```python
from build123d import *

# Parameters (mm, degrees)
F1_DEPTH       = 180
F3_D           = 4.5
F3_CBORE_D     = 8.5
F3_CBORE_DEPTH = 5.5


with BuildPart() as f1:
    # F0 (on Right) → F1 (new body)
    with BuildSketch(Plane.YZ):
        with BuildLine():
            Line((-6.8, 0), (6.8, 0))
            Line((6.8, 0), (7.5, 0.7))
            Line((7.5, 0.7), (7.5, 3.699439))
            Line((7.5, 3.699439), (4.799805, 6.399634))
            Line((4.799805, 6.399634), (4.799805, 8.409149))
            Line((4.799805, 8.409149), (5.200758, 8.810103))
            ThreePointArc((5.200758, 8.810103), (5.668922, 9.789262), (6.648081, 10.257425))
            Line((6.648081, 10.257425), (7.5, 11.109345))
            Line((7.5, 11.109345), (7.5, 12.449454))
            Line((7.5, 12.449454), (6.634491, 13.314965))
            ThreePointArc((6.634491, 13.314965), (5.668922, 13.781617), (5.20227, 14.747186))
            Line((5.20227, 14.747186), (4.949456, 15))
            Line((4.949456, 15), (-4.949456, 15))
            Line((-4.949456, 15), (-5.20227, 14.747186))
            ThreePointArc((-5.20227, 14.747186), (-5.668922, 13.781617), (-6.634491, 13.314965))
            Line((-6.634491, 13.314965), (-7.5, 12.449454))
            Line((-7.5, 12.449454), (-7.5, 11.109345))
            Line((-7.5, 11.109345), (-6.648081, 10.257425))
            ThreePointArc((-6.648081, 10.257425), (-5.668922, 9.789262), (-5.200758, 8.810103))
            Line((-5.200758, 8.810103), (-4.799805, 8.409149))
            Line((-4.799805, 8.409149), (-4.799805, 6.399634))
            Line((-4.799805, 6.399634), (-7.5, 3.699439))
            Line((-7.5, 3.699439), (-7.5, 0.7))
            Line((-7.5, 0.7), (-6.8, 0))
        make_face()
    extrude(amount=F1_DEPTH)

    # F3 (through all)
    with Locations(Plane.XY.offset(15)):
        with Locations((6.75, 0), (62.25, 0), (117.75, 0), (173.25, 0)):
            CounterBoreHole(F3_D / 2, F3_CBORE_D / 2, F3_CBORE_DEPTH)


solid = f1.part
```
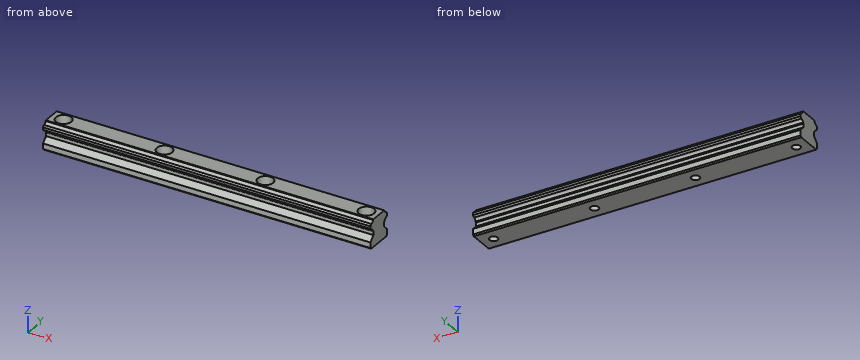
For this review, take the finished solid that the model builds, in its own axes (mm). Round coordinates to 2 decimals unless told otherwise and drop trailing zeros. Write each loop counter-clockwise with the first axis right and the second up, starting at its lowest first coordinate (ties: lowest second). Pieces come first, ordered by that corner, then holes. Notation, with made-up numbers: (2, 0) - (15, 0) arc R32 cw to (15, 30) - close; hole circle Ø5 at (32, -9). An arc over 180 degrees is marked (long way). Answer as a JSON object with one key per item and string values.
1. We need section C-C on y = 0. Count the separate pieces of the cut face and the enclosed holes in it, then the cut area to 3 significant figures.
Response values:
{"separate pieces": "5", "enclosed holes": "0", "area": "2,340 mm2"}
2. To check wall thickness, follow line 1 along X through (y, z) = (-1.5, 12); line 2 along Y through (x, z) = (117.75, 2.75); line 3 along X through (y, z) = (2.5, 14.5). State the ranges of each line that lie inside material, in increasing order.
Response values:
{"line 1": "x = 0 to 2.77, 10.73 to 58.27, 66.23 to 113.77, 121.73 to 169.27, 177.23 to 180", "line 2": "y = -7.5 to -2.25, 2.25 to 7.5", "line 3": "x = 0 to 3.31, 10.19 to 58.81, 65.69 to 114.31, 121.19 to 169.81, 176.69 to 180"}
3. For pin 1 Ø5 at (x, y) = (117.75, 0) entering from +Z; pin 2 Ø4 at (x, z) = (43, 7.5) entering from +Y; pin 3 Ø1 at (x, z) = (66, 7.5) entering from -Y, all flat-tipped, find the tip position at first contact; note any pin that passes through.
Response values:
{"pin 1": "stops at z = 9.5", "pin 2": "stops at y = 5.7", "pin 3": "stops at y = -4.8"}
4. We need section B-B on x = 144. Give the boundary of the cut face in (y, z).
Response values:
{"outline": "(-7.5, 0.7) - (-6.8, 0) - (6.8, 0) - (7.5, 0.7) - (7.5, 3.7) - (4.8, 6.4) - (4.8, 8.41) - (5.2, 8.81) arc R1.63 cw to (6.65, 10.26) - (7.5, 11.11) - (7.5, 12.45) - (6.63, 13.31) arc R1.63 cw to (5.2, 14.75) - (4.95, 15) - (-4.95, 15) - (-5.2, 14.75) arc R1.63 cw to (-6.63, 13.31) - (-7.5, 12.45) - (-7.5, 11.11) - (-6.65, 10.26) arc R1.63 cw to (-5.2, 8.81) - (-4.8, 8.41) - (-4.8, 6.4) - (-7.5, 3.7) - close"}
